```python
from build123d import *

# Parameters (mm, degrees)
F0_W     = 228.6
F0_H     = 152.4
F1_DEPTH = 152.4
F2_W     = 76.2
F2_H     = 127
F3_DEPTH = 76.2
F4_W     = 50.793443
F4_H     = 52.342028
F5_DEPTH = 25.4
F6_R     = 25.4


with BuildPart() as f1:
    # F0 (on Front) → F1 (new body)
    with BuildSketch(Plane.XZ):
        with Locations((-114.3, 76.2)):
            Rectangle(F0_W, F0_H)
    extrude(amount=F1_DEPTH)

    # F2 (on face) → F3 (cut)
    with BuildSketch(Plane.XZ.offset(152.4)):
        with Locations((-114.3, 88.9)):
            Rectangle(F2_W, F2_H)
    extrude(amount=-F3_DEPTH, mode=Mode.SUBTRACT)

    # F4 (on face) → F5 (cut)
    with BuildSketch(Plane.YZ):
        with Locations((-75.265935, 79.911679)):
            Rectangle(F4_W, F4_H)
    extrude(amount=-F5_DEPTH, mode=Mode.SUBTRACT)

    # F6
    f6_edges = [f1.edges().sort_by_distance(p)[0] for p in [
        (0, 0, 76.2),
    ]]
    fillet(f6_edges, radius=F6_R)


solid = f1.part
```
Verification items for the finished model (mm, model axes). A direction names the side the tool comes from. Give positions to 0.01 mm unless a question says otherwise; leave off trailing zeros. Write each loop counter-clockwise with the first axis right and the second up, starting at its lowest first coordinate (ties: lowest second). Pieces come first, ordered by that corner, then holes. Notation, with made-up numbers: M 42,8 L 75,8 A28 cw 75,39 Z; hole C 14,50.5 d3. An arc over 180 degrees is marked long. One line per question, with ' | ' between items.
1) Section check C-C on x = -145.5. Enter the section's corners in (y, z), plus the area to 3 significant figures.
Result:
outline: M -152.4,0 L 0,0 L 0,152.4 L -76.2,152.4 L -76.2,25.4 L -152.4,25.4 Z | area: 13,500 mm2
2) Mould release check, pull along Y, two halves, no side actions. Record for faces 4 (the flat face through (-128, 0, 77)), 5 (the flat face through (-13, -49.869, 80)), 6 (the flat face through (0, -102, 75)): released by +Y, released by -Y, zero draft, split by the parting line, or undercut.
Result:
face 4: released by +Y | face 5: undercut | face 6: zero draft
3) Thickness scan on line 1 along X through (y, z) = (-137, 93.5); line 2 along Z through (x, y) = (-15, -98.5); line 3 along X through (y, z) = (-89.5, 97). Record the ranges inside material, lowest first. Write a range as [from, to].
Result:
line 1: x = [-228.6, -152.4], [-76.2, 0] | line 2: z = [0, 53.74], [106.08, 152.4] | line 3: x = [-228.6, -152.4], [-76.2, -25.4]
4) Section check A-A on y = -122. Enter the section's corners in (x, z), plus the area to 3 significant figures.
Result:
outline: M -228.6,0 L 0,0 L 0,152.4 L -76.2,152.4 L -76.2,25.4 L -152.4,25.4 L -152.4,152.4 L -228.6,152.4 Z | area: 25,200 mm2
5) Section check B-B on z = 80. Enter the section's corners in (x, y).
Result:
outline: M -228.6,-152.4 L -152.4,-152.4 L -152.4,-76.2 L -76.2,-76.2 L -76.2,-152.4 L 0,-152.4 L 0,-100.66 L -25.4,-100.66 L -25.4,-49.87 L 0,-49.87 L 0,-25.4 A25.4 ccw -25.4,0 L -228.6,0 Z
6) Gauge pin test, flat end, axial feed: pin 1 Ø20.5 at (x, z) = (-11, 74.5) entering from +Y. Record the tip position at first contact, or that the pin passes through.
Result:
pin 1: stops at y = -0.34
7) Set-up check for faces 1 (the cylindrical face through (-7.64, -7.24, 77.27)), 2 (the flat face through (-13, -76, 106.083)), 3 (the flat face through (-152.4, -115, 88)): record each of +Z, -Z, +X, -X, +Y, -Y from which the full face is reachable in a straight line by a thin tool's end or side.
Result:
face 1: +Z, -Z, +X, +Y | face 2: +X | face 3: +Z, -Y
8) Section check D-D on z = 131.5. Enter the section's corners in (x, y).
Result:
outline: M -228.6,-152.4 L -152.4,-152.4 L -152.4,-76.2 L -76.2,-76.2 L -76.2,-152.4 L 0,-152.4 L 0,-25.4 A25.4 ccw -25.4,0 L -228.6,0 Z
